The model under review builds one solid part; all positions refer to its coordinate system, in mm. Coordinates: 2 decimals unless noted, no trailing zeros. Write each loop counter-clockwise with the first axis right and the second up, starting at its lowest first coordinate (ties: lowest second). Pieces come first, ordered by that corner, then holes.
```python
from build123d import *

# Parameters (mm, degrees)
SKETCH_1_R          = 8.75
EXTRUDE_1_DEPTH     = 10
CUT_EXTRUDE_1_REACH = 17.91
SKETCH_2_R          = 6.25
EXTRUDE_START       = 1
SKETCH_3_R          = 7
SKETCH_3_R_2        = 6.25
EXTRUDE_2_DEPTH     = 1
SKETCH_4_R          = 7
SKETCH_4_R_2        = 6.25
EXTRUDE_3_DEPTH     = 1


with BuildPart() as part:
    # 草图1 → 凸台-拉伸1 (new body)
    with BuildSketch(Plane(origin=(0, 0, 0), x_dir=(1, 0, 0), z_dir=(0, 1, 0))):
        with Locations(Location((0, 0, 0), (0, 0, 270))):
            Circle(SKETCH_1_R)
    extrude(amount=EXTRUDE_1_DEPTH)

    # 草图2 → 切除-拉伸1 (cut, up to next)
    with BuildSketch(Plane(origin=(0, 10, 0), x_dir=(1, 0, 0), z_dir=(0, 1, 0)), mode=Mode.PRIVATE) as cut_extrude_1_sk1:
        with Locations(Location((0, 0, 0), (0, 0, 270))):
            Circle(SKETCH_2_R)
    cut_extrude_1_tool1 = extrude(cut_extrude_1_sk1.sketch, amount=-CUT_EXTRUDE_1_REACH, mode=Mode.PRIVATE) & part.part
    add(cut_extrude_1_tool1.solids().sort_by_distance((0, 10, 0))[0], mode=Mode.SUBTRACT)

    # 草图3 → 凸台-拉伸2 (add)
    with BuildSketch(Plane(origin=(0, 10, 0), x_dir=(1, 0, 0), z_dir=(0, 1, 0)).offset(EXTRUDE_START)):
        with Locations(Location((0, 0, 0), (0, 0, 270))):
            Circle(SKETCH_3_R)
        with Locations(Location((0, 0, 0), (0, 0, 270))):
            Circle(SKETCH_3_R_2, mode=Mode.SUBTRACT)
    extrude(amount=-EXTRUDE_2_DEPTH)

    # 草图4 → 凸台-拉伸3 (add)
    with BuildSketch(Plane.XZ):
        with Locations(Location((0, 0, 0), (0, 0, 90))):
            Circle(SKETCH_4_R)
        with Locations(Location((0, 0, 0), (0, 0, 90))):
            Circle(SKETCH_4_R_2, mode=Mode.SUBTRACT)
    extrude(amount=EXTRUDE_3_DEPTH)

    # 草图5 → 旋转1 (revolve)
    with BuildSketch(Plane.XY, mode=Mode.PRIVATE) as revolve_1_sk:
        Polygon((-7, 11), (-8.75, 10), (-7, 10), align=None)
        Polygon((-8.75, 0), (-7, 0), (-7, -1), align=None)
    revolve(revolve_1_sk.sketch.rotate(Axis((0, 12.096395085, 0), (0, -1, 0)), 270), axis=Axis((0, 12.096395085, 0), (0, -1, 0)))


solid = part.part
```
Item 1: Mouldability with a two-part tool opening along Z and no side actions: class faces 1 (the face through (6, 11, -3)), 2 (the face through (-5.324, 4.93, -6.944)), 3 (the face through (-1.88, 5.08, 5.96)) as pulls with the +Z half, pulls with the -Z half, needs draft (parallel to the pull), parting line crosses it, or undercut.
Solved:
face 1: needs draft
face 2: parting line crosses it
face 3: undercut
Item 2: To check wall thickness, follow line 1 along X through (y, z) = (7, 0); line 2 along Z through (x, y) = (4.5, 5.5); line 3 along Z through (x, y) = (-5.25, 2.5). State the ranges of each line that lie inside material, in increasing order.
Solved:
line 1: x = -8.75 to -6.25, 6.25 to 8.75
line 2: z = -7.5 to -4.34, 4.34 to 7.5
line 3: z = -7 to -3.39, 3.39 to 7
Item 3: Take a section at A-A, the plane z = 0. Write out the cut boundary in (x, y), plus the area to 3 significant figures.
Solved:
outline: (-8.75, 0) - (-7, -1) - (-6.25, -1) - (-6.25, 11) - (-7, 11) - (-8.75, 10) - close; (6.25, -1) - (7, -1) - (8.75, 0) - (8.75, 10) - (7, 11) - (6.25, 11) - close
area: 56.5 mm2
Item 4: Take a section at C-C, the plane y = 2.75. Write out the cut boundary in (x, z).
Solved:
outline: circle Ø17.5 at (0, 0); hole circle Ø12.5 at (0, 0)
Item 5: For pin 1 (4 mm diameter, centred on x = 2, y = 2, fed in from +Z); pin 2 (3 mm diameter, centred on y = 9.5, z = -4, fed in from +X); pin 3 (4 mm diameter, centred on y = 1.5, z = 5, fed in from +X); pin 4 (5 mm diameter, centred on x = 5.5, y = 7, fed in from -Z), all flat-tipped, find the tip position at first contact; note any pin that passes through.
Solved:
pin 1: stops at z = 8.75
pin 2: stops at x = 8.39
pin 3: stops at x = 8.22
pin 4: stops at z = -8.22
Item 6: Take a section at B-B, the plane x = 0. Write out the cut boundary in (y, z).
Solved:
outline: (-1, -7) - (0, -8.75) - (10, -8.75) - (11, -7) - (11, -6.25) - (-1, -6.25) - close; (-1, 6.25) - (11, 6.25) - (11, 7) - (10, 8.75) - (0, 8.75) - (-1, 7) - close
